Read the model definition and answer for the solid it produces. Units are mm, in the model's axes. Give positions to 0.01 mm unless a question says otherwise; leave off trailing zeros. Order: outer loops, then holes, each group sorted by start corner. A loop starts at its lowest first (then second) coordinate and runs counter-clockwise, first axis right, second up. Notation, with made-up numbers: (-28.5, -8) - (-7.5, -8) arc R4 cw to (-7.5, -2) - close; hole circle Ø2 at (24, -17). An arc over 180 degrees is marked (long way). Return JSON: item names as keys, results as strings.
```python
from build123d import *

# Parameters (mm, degrees)
SKETCH1_W           = 198
SKETCH1_H           = 88
BOSS_EXTRUDE1_DEPTH = 4
SKETCH2_R           = 2.1
CUT_EXTRUDE1_DEPTH  = 217.711790173
SKETCH3_R           = 2
CUT_EXTRUDE2_DEPTH  = 10
SKETCH4_R           = 2
CUT_EXTRUDE3_DEPTH  = 25


with BuildPart() as part:
    # Sketch1 → Boss-Extrude1 (new body)
    with BuildSketch(Plane(origin=(0, 0, 0), x_dir=(1, 0, 0), z_dir=(0, 1, 0))):
        with Locations((99, 44)):
            Rectangle(SKETCH1_W, SKETCH1_H)
    extrude(amount=BOSS_EXTRUDE1_DEPTH)

    # Sketch2 → Cut-Extrude1 (cut, through all)
    with BuildSketch(Plane.XZ):
        with Locations(Location((12.5, -26.25, 0), (0, 0, 270))):
            Circle(SKETCH2_R)
        with Locations(Location((69.5, -26.25, 0), (0, 0, 270))):
            Circle(SKETCH2_R)
        with Locations(Location((69.5, -70.75, 0), (0, 0, 270))):
            Circle(SKETCH2_R)
        with Locations(Location((12.5, -70.75, 0), (0, 0, 270))):
            Circle(SKETCH2_R)
    extrude(amount=-CUT_EXTRUDE1_DEPTH, mode=Mode.SUBTRACT)

    # Sketch3 → Cut-Extrude2 (cut)
    with BuildSketch(Plane.XZ):
        with Locations(Location((30, -79.91533843, 0), (0, 0, 270))):
            Circle(SKETCH3_R)
        with Locations(Location((168, -79.91533843, 0), (0, 0, 270))):
            Circle(SKETCH3_R)
    extrude(amount=-CUT_EXTRUDE2_DEPTH, mode=Mode.SUBTRACT)

    # Sketch4 → Cut-Extrude3 (cut)
    with BuildSketch(Plane.XZ):
        with Locations(Location((7, -44, 0), (0, 0, 270))):
            Circle(SKETCH4_R)
        with Locations(Location((191, -44, 0), (0, 0, 270))):
            Circle(SKETCH4_R)
    extrude(amount=-CUT_EXTRUDE3_DEPTH, mode=Mode.SUBTRACT)


solid = part.part
```
Q1. Determine the mould class of faces 1 (the cylindrical face through (68.2, 2, -24.6)), 2 (the flat face through (98, 0, -45)), 3 (the flat face through (198, 2, -43)) for opening direction X: released by +X, released by -X, zero draft, split by the parting line, or undercut.
Values:
{"face 1": "undercut", "face 2": "zero draft", "face 3": "released by +X"}
Q2. A cutting plane is placed at A-A (x = 69.5). Write down the section's boundary in (y, z).
Values:
{"outline": "(0, -88) - (4, -88) - (4, -72.85) - (0, -72.85) - close; (0, -68.65) - (4, -68.65) - (4, -28.35) - (0, -28.35) - close; (0, -24.15) - (4, -24.15) - (4, 0) - (0, 0) - close"}
Q3. A cutting plane is placed at B-B (z = -70.75). Write down the section's boundary in (x, y).
Values:
{"outline": "(0, 0) - (10.4, 0) - (10.4, 4) - (0, 4) - close; (14.6, 0) - (67.4, 0) - (67.4, 4) - (14.6, 4) - close; (71.6, 0) - (198, 0) - (198, 4) - (71.6, 4) - close"}
Q4. A cutting plane is placed at C-C (x = 168). Write down the section's boundary in (y, z).
Values:
{"outline": "(0, -88) - (4, -88) - (4, -81.92) - (0, -81.92) - close; (0, -77.92) - (4, -77.92) - (4, 0) - (0, 0) - close"}
Q5. Consider L1, parallel to X at y = 2.15, z = -44; L2, parallel to X at y = 2.2, z = -70.75; L3, parallel to Z at x = 191, y = 1.25. Determine where each line is inside the solid, lowest interval first.
Values:
{"L1": "x = 0 to 5, 9 to 189, 193 to 198", "L2": "x = 0 to 10.4, 14.6 to 67.4, 71.6 to 198", "L3": "z = -88 to -46, -42 to 0"}
Q6. Given pin 1 (2.5 mm diameter, centred on x = 69.5, z = -70.75, fed in from +Y), flat-ended and moving along its own axis, determine where the tip first touches the part or whether it passes through.
Values:
{"pin 1": "passes through"}
